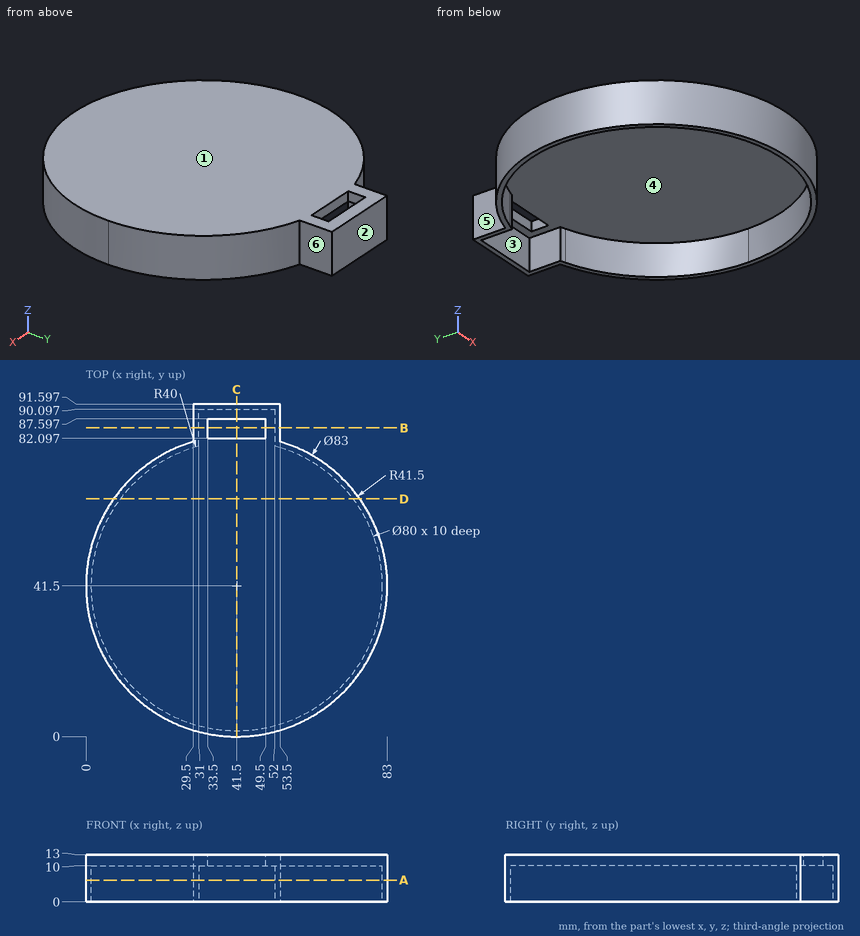
Input: dimensioned drawing with shaded views. Units: mm. Origin: part minimum x, y, z. A direction names the side the tool comes from. Give positions to 0.01 mm unless a question says otherwise; leave off trailing zeros. Order: outer loops, then holes, each group sorted by start corner. A loop starts at its lowest first (then second) coordinate and runs counter-clockwise, first axis right, second up.
(1) Pull-direction query (Y, two-part tool) for the marked faces 1, 2 and 3; classes: +Y half, -Y half, draft (parallel to the pull), parting line (faces both ways), or undercut.
(2) Contact query for flat-ended pins moving along their axis: P1, Ø2, axis at x = 35, z = 9.5, coming from the -Y side; P2, Ø2.5, axis at y = 85.5, z = 12, coming from the +X side; P3, Ø1.5, axis at x = 69, y = 41.5, coming from the -Z side. Output: stop coordinate, or through.
(3) Section query A-A (z = 6). Return the cut outline in (x, y), plus the area to 3 significant figures.
(4) Section query B-B (y = 85). Return the cut outline in (x, z), plus the area to 3 significant figures.
(5) Section query D-D (y = 65.5). Return the cut outline in (x, z), plus the area to 3 significant figures.
(6) Access query for the marked faces 4, 5 and 6. Directions: +Z, -Z, +X, -X, +Y, -Y. A direction counts if a zero-diameter tool reaches every point of the face in a straight line with its end or side. Return the directions, or none.
(7) Material intervals for line 1 along X through (y, z) = (41.5, 8.25); line 2 along Y through (x, z) = (41.5, 2); line 3 along Z through (x, y) = (56.5, 47.5), sorted ascending.
(8) Section query C-C (x = 41.5). Return the cut outline in (y, z), plus the area to 3 significant figures.
Outcome:
1. face 1: draft
1. face 2: +Y half
1. face 3: undercut
2. P1: stops at y = 0.37
2. P2: stops at x = 53.5
2. P3: stops at z = 10
3. outline: (29.5, 81.23) arc R41.5 ccw (long way) to (53.5, 81.23) - (53.5, 91.6) - (29.5, 91.6) - close; hole (31, 80.1) arc R40 ccw (long way) to (52, 80.1) - (52, 90.1) - (31, 90.1) - close
3. area: 414 mm2
4. outline: (29.5, 0) - (31, 0) - (31, 10) - (33.5, 10) - (33.5, 13) - (29.5, 13) - close; (49.5, 10) - (52, 10) - (52, 0) - (53.5, 0) - (53.5, 13) - (49.5, 13) - close
4. area: 54.0 mm2
5. outline: (7.64, 0) - (9.5, 0) - (9.5, 10) - (73.5, 10) - (73.5, 0) - (75.36, 0) - (75.36, 13) - (7.64, 13) - close
5. area: 240 mm2
6. face 4: -Z
6. face 5: +Z, -Z, -X, +Y
6. face 6: +Z, -Z, +X, +Y
7. line 1: x = 0 to 1.5, 81.5 to 83
7. line 2: y = 0 to 1.5, 90.1 to 91.6
7. line 3: z = 10 to 13
8. outline: (0, 0) - (1.5, 0) - (1.5, 10) - (82.1, 10) - (82.1, 13) - (0, 13) - close; (87.6, 10) - (90.1, 10) - (90.1, 0) - (91.6, 0) - (91.6, 13) - (87.6, 13) - close
8. area: 288 mm2
